```python
from build123d import *

# Parameters (mm, degrees)
SKETCH2_R          = 1.5
CUT_EXTRUDE5_DEPTH = 24.452078799


with BuildPart() as part:
    # Sketch1 → Revolve1 (revolve)
    with BuildSketch(Plane.XY, mode=Mode.PRIVATE) as revolve1_sk:
        Polygon((10, 4), (3, 4), (3, 15), (0, 15), (0, 2), (10, 2), align=None)
    revolve(revolve1_sk.sketch.rotate(Axis((0, 0, 0), (1, 0, 0)), 90), axis=Axis((0, 0, 0), (1, 0, 0)))

    # Sketch2 → Cut-Extrude5 (cut, through all)
    with BuildSketch(Plane.ZY):
        with Locations((0, 10.5)):
            Circle(SKETCH2_R)
        with Locations((9.09326674, 5.25)):
            Circle(SKETCH2_R)
        with Locations((9.09326674, -5.25)):
            Circle(SKETCH2_R)
        with Locations((0, -10.5)):
            Circle(SKETCH2_R)
        with Locations((-9.09326674, -5.25)):
            Circle(SKETCH2_R)
        with Locations((-9.09326674, 5.25)):
            Circle(SKETCH2_R)
    extrude(amount=-CUT_EXTRUDE5_DEPTH, mode=Mode.SUBTRACT)


solid = part.part
```
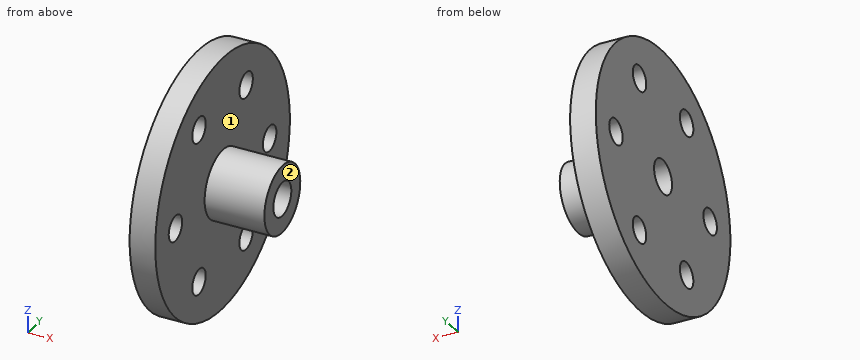
Part model, mm, in its own coordinate system. Face numbers are marked on the shaded views. A direction names the side the tool comes from. Round coordinates to 2 decimals unless told otherwise and drop trailing zeros. Order: outer loops, then holes, each group sorted by start corner. A loop starts at its lowest first (then second) coordinate and runs counter-clockwise, first axis right, second up. Notation, with made-up numbers: M 66,-17.5 L 70,-17.5 A27 cw 70,4.5 Z; hole C 77,-23 d7. An arc over 180 degrees is marked long. Put each result on its own line as item: value. Start each with the question number.
1. Slice it at A-A on x = 2. List the corners of the cut face in (y, z).
2. Slice it at C-C on z = 0. List the corners of the cut face in (x, y), then the cut area to 3 significant figures.
3. Slice it at D-D on y = -10.5. List the corners of the cut face in (x, z), then the cut area to 3 significant figures.
4. Drop flat-ended pins along their axis: pin 1 (5 mm diameter, centred on x = 7, y = 9, fed in from +Z); pin 2 (2 mm diameter, centred on x = 6.5, z = -1.5, fed in from +Y); pin 3 (4 mm diameter, centred on y = 5.25, z = -9.09, fed in from +X); pin 4 (6 mm diameter, centred on x = 3, y = -12, fed in from +Z). Give the stop position or say it passes through.
5. Drill centre lines: probe 1 along Y at (x, z) = (2.3, 0); probe 2 along Y at (x, z) = (1, 9); probe 3 along X at (y, z) = (10.5, 3.25). Where is each one in solid material? Low to high. Write a range as [from, to].
6. Tool access for the marked faces 1 and 2: list every direction of +Z, -Z, +X, -X, +Y, -Y with a clear straight run to the whole face (end or side of a thin tool).
7. Slice it at B-B on y = 4.75. List the corners of the cut face in (x, z), then the cut area to 3 significant figures.
Findings:
1. outline: C 0,0 d30; hole C -10.5,0 d3; hole C -5.25,-9.09 d3; hole C -5.25,9.09 d3; hole C 0,0 d4; hole C 5.25,-9.09 d3; hole C 5.25,9.09 d3; hole C 10.5,0 d3
2. outline: M 0,-15 L 3,-15 L 3,-12 L 0,-12 Z; M 0,-9 L 3,-9 L 3,-4 L 10,-4 L 10,-2 L 0,-2 Z; M 0,2 L 10,2 L 10,4 L 3,4 L 3,9 L 0,9 Z; M 0,12 L 3,12 L 3,15 L 0,15 Z
2. area: 88.0 mm2
3. outline: M 0,-10.71 L 3,-10.71 L 3,-1.5 L 0,-1.5 Z; M 0,1.5 L 3,1.5 L 3,10.71 L 0,10.71 Z
3. area: 55.3 mm2
4. pin 1: through
4. pin 2: y = 3.97
4. pin 3: x = 3
4. pin 4: z = 12
5. probe 1: [-15, -12], [-9, -2], [2, 9], [12, 15]
5. probe 2: [-12, -6.75], [-3.75, 3.75], [6.75, 12]
5. probe 3: [0, 3]
6. face 1: +X
6. face 2: +Z, -Z, +X, +Y, -Y
7. outline: M 0,-14.23 L 3,-14.23 L 3,-10.51 L 0,-10.51 Z; M 0,-7.68 L 3,-7.68 L 3,7.68 L 0,7.68 Z; M 0,10.51 L 3,10.51 L 3,14.23 L 0,14.23 Z
7. area: 68.4 mm2
